Source: CAD feature listing. Evaluate the final solid. Frame: model axes, mm. A direction names the side the tool comes from. Give positions to 0.01 mm unless a question says otherwise; leave off trailing zeros. Loops run counter-clockwise (first coordinate to the right, second up) from the corner with the lowest first, then second, coordinate; pieces in that order, holes last. Notation, with made-up numbers: (-8.75, 67) -> (41.25, 67) arc R29 cw to (41.25, 92) -> close; hole circle Ø6 at (-1, -3). An arc over 180 degrees is marked (long way). Return JSON: item names as keys, results as strings. Group by question number.
```python
from build123d import *

# Parameters (mm, degrees)
MODEL_R                        = 20.5
MODEL_R_2                      = 0.75
MAIN_DIFFERENTIAL_DISK_DEPTH   = 4
TENDON_HOLDER_DEPTH            = 5
DIFFERENTIAL_DISK_CONTOURING_R = 0.2


with BuildPart() as part:
    # Model → Main Differential Disk (new body)
    with BuildSketch(Plane.XY):
        Circle(MODEL_R)
        with Locations((-8.75, 15.155444566)):
            Circle(MODEL_R_2, mode=Mode.SUBTRACT)
        with Locations((8.75, 15.155444566)):
            Circle(MODEL_R_2, mode=Mode.SUBTRACT)
        with Locations((17.5, 0)):
            Circle(MODEL_R_2, mode=Mode.SUBTRACT)
        with Locations((8.75, -15.155444566)):
            Circle(MODEL_R_2, mode=Mode.SUBTRACT)
        with Locations((-8.75, -15.155444566)):
            Circle(MODEL_R_2, mode=Mode.SUBTRACT)
        Circle(MODEL_R_2, mode=Mode.SUBTRACT)
        with Locations((-17.5, 0)):
            Circle(MODEL_R_2, mode=Mode.SUBTRACT)
    extrude(amount=MAIN_DIFFERENTIAL_DISK_DEPTH)

    # Sketch1 → Tendon Holder (cut, through all)
    with BuildSketch(Plane.XY.offset(4)):
        with BuildLine():
            Line((-18.25, 0), (-20.121847663, 3.919342625))
            ThreePointArc((-20.121847663, 3.919342625), (-19.953970316, 4.699900916), (-19.755825892, 5.473330187))
            Line((-19.755825892, 5.473330187), (-17.5, 0.75))
            ThreePointArc((-17.5, 0.75), (-16.969669914, -0.530330086), (-18.25, 0))
        make_face()
        with BuildLine():
            Line((-9.125, 15.804963619), (-6.666673552, 19.38570256))
            ThreePointArc((-6.666673552, 19.38570256), (-5.906751569, 19.630595658), (-5.137869961, 19.845712188))
            Line((-5.137869961, 19.845712188), (-8.100480947, 15.530444566))
            ThreePointArc((-8.100480947, 15.530444566), (-8.944114284, 14.431000197), (-9.125, 15.804963619))
        make_face()
        with BuildLine():
            Line((9.125, 15.804963619), (13.455174111, 15.466359935))
            ThreePointArc((13.455174111, 15.466359935), (14.047218747, 14.930694742), (14.617955931, 14.372382002))
            Line((14.617955931, 14.372382002), (9.399519053, 14.780444566))
            ThreePointArc((9.399519053, 14.780444566), (8.02555563, 14.961330282), (9.125, 15.804963619))
        make_face()
        with BuildLine():
            Line((18.25, 0), (20.121847663, -3.919342625))
            ThreePointArc((20.121847663, -3.919342625), (19.953970316, -4.699900916), (19.755825892, -5.473330187))
            Line((19.755825892, -5.473330187), (17.5, -0.75))
            ThreePointArc((17.5, -0.75), (16.969669914, 0.530330086), (18.25, 0))
        make_face()
        with BuildLine():
            Line((9.125, -15.804963619), (6.666673552, -19.38570256))
            ThreePointArc((6.666673552, -19.38570256), (5.906751569, -19.630595658), (5.137869961, -19.845712188))
            Line((5.137869961, -19.845712188), (8.100480947, -15.530444566))
            ThreePointArc((8.100480947, -15.530444566), (8.944114284, -14.431000197), (9.125, -15.804963619))
        make_face()
        with BuildLine():
            Line((-9.125, -15.804963619), (-13.455174111, -15.466359935))
            ThreePointArc((-13.455174111, -15.466359935), (-14.047218747, -14.930694742), (-14.617955931, -14.372382002))
            Line((-14.617955931, -14.372382002), (-9.399519053, -14.780444566))
            ThreePointArc((-9.399519053, -14.780444566), (-8.02555563, -14.961330282), (-9.125, -15.804963619))
        make_face()
    extrude(amount=-TENDON_HOLDER_DEPTH, mode=Mode.SUBTRACT)

    # Differential Disk Contouring
    differential_disk_contouring_edges = [part.edges().sort_by_distance(p)[0] for p in [
        (6.666673552, -19.38570256, 2),
        (-13.455174111, -15.466359935, 2),
        (-20.121847663, 3.919342625, 2),
        (-6.666673552, 19.38570256, 2),
        (13.455174111, 15.466359935, 2),
        (20.121847663, -3.919342625, 2),
    ]]
    fillet(differential_disk_contouring_edges, radius=DIFFERENTIAL_DISK_CONTOURING_R)


solid = part.part
```
1) Cut plane C-C on y = 10. Return loops of the section in (x, z).
2) Cut plane D-D on x = -10.5. Return loops of the section in (y, z).
3) Cut plane A-A on x = 0. Return loops of the section in (y, z).
4) Reachability of faces 1 (the face through (12.045, 14.574, 2.028)), 2 (the face through (-12.045, -14.574, 2.028)), 3 (the face through (-18.64, 3.14, 2.03)), 4 (the face through (0, -4, 4)) from +Z, -Z, +X, -X, +Y, -Y: full face, straight path, thin tool, end or side. Return the list, or none.
5) Mould query, pull axis Y, two halves, no side actions, for faces 5 (the face through (15.05, -13.92, 1.97)), 6 (the face through (10.954, 15.662, 2.028)), 7 (the face through (-15.05, 13.92, 1.97)), 8 (the face through (-16.99, -0.55, 1.97)). Classes: released by +Y, released by -Y, zero draft, split by the parting line, or undercut.
6) Material intervals for line 1 (Y direction, x = 8.75, z = 1.75); line 2 (Y direction, x = -7.5, z = 0.5); line 3 (Y direction, x = 0, z = 1), sorted ascending.
Calculated:
{
 "1": {"outline": "(-17.9, 0) -> (17.9, 0) -> (17.9, 4) -> (-17.9, 4) -> close"},
 "2": {"outline": "(-17.61, 0) -> (-15.7, 0) -> (-15.7, 4) -> (-17.61, 4) -> close; (-14.69, 0) -> (17.61, 0) -> (17.61, 4) -> (-14.69, 4) -> close"},
 "3": {"outline": "(-20.5, 0) -> (-0.75, 0) -> (-0.75, 4) -> (-20.5, 4) -> close; (0.75, 0) -> (20.5, 0) -> (20.5, 4) -> (0.75, 4) -> close"},
 "4": {"face 1": "+Z, -Z, +X", "face 2": "+Z, -Z, -X", "face 3": "+Z, -Z", "face 4": "+Z, +X, -X, +Y, -Y"},
 "5": {"face 5": "released by -Y", "face 6": "undercut", "face 7": "released by +Y", "face 8": "undercut"},
 "6": {"line 1": "-18.54 to -16.35, -14.41 to 14.41, 15.91 to 18.54", "line 2": "-19.08 to 16.41, 18.17 to 19.08", "line 3": "-20.5 to -0.75, 0.75 to 20.5"}
}
